CAD build for the part. Positions are in the model's coordinates, mm. A direction names the side the tool comes from. Round coordinates to 2 decimals unless told otherwise and drop trailing zeros. Write each loop counter-clockwise with the first axis right and the second up, starting at its lowest first coordinate (ties: lowest second). Pieces come first, ordered by that corner, then holes. Notation, with made-up numbers: (68.5, 23) -> (101.5, 23) arc R16 ccw to (101.5, 32) -> close; hole circle Ø8 at (88, 9). An arc over 180 degrees is marked (long way). Put each result on its own line as item: value. Start each with the question number.
1. Drill centre lines: line 1 (X direction, y = 7, z = -9); line 2 (Z direction, x = 2, y = 3.5); line 3 (Y direction, x = -4.5, z = 10). Where is each one in solid material? Low to high. Write a range as from..to.
2. Saw through at B-B on x = 5. List the corners of the cut face in (y, z).
3. 3-axis set-ups, long thin cutter, end or side, ignore diameter. For faces 4 (the flat face through (17, 0, -23)), 5 (the flat face through (13.79, 4, 2)), 6 (the flat face through (-32, -1, -26.874)), 7 (the flat face through (17, -1, 24.126)), 8 (the cylindrical face through (-34.64, -0.99, 24.73)): which of +Z, -Z, +X, -X, +Y, -Y reach the whole face in a straight line?
4. Saw through at C-C on z = -10.5. List the corners of the cut face in (x, y).
5. Pull direction Z, two halves, no side cores. Call faces 1 (the cylindrical face through (20.22, -0.986, 28.524)), 2 (the cylindrical face through (-34.64, -0.99, -26.27)), 3 (the cylindrical face through (20.22, -0.986, -22.476)): pulls with the +Z half, pulls with the -Z half, needs draft (parallel to the pull), parting line crosses it, or undercut.
6. Flat gauge pins, fed straight in: P1, Ø0.6, axis at x = -32, y = -0.5, coming from the -Z side; P2, Ø2, axis at x = 17.5, y = -0.5, coming from the +Z side; P3, Ø1.5, axis at y = -0.5, z = 4, coming from the -X side; P4, Ø4, axis at x = -32.71, z = 26.63, coming from the -Y side. Where does each tip first touch, or does it go through?
7. Saw through at A-A on y = 2.25. List the corners of the cut face in (x, z).
from build123d import *

# Parameters (mm, degrees)
SKETCH_1_W          = 46
SKETCH_1_H          = 62
EXTRUDE_1_DEPTH     = 8
SKETCH_2_W          = 42
SKETCH_2_H          = 58
CUT_EXTRUDE_1_DEPTH = 8
SKETCH_3_R          = 1.5
SKETCH_3_W          = 42
SKETCH_3_H          = 58
EXTRUDE_2_DEPTH     = 2


with BuildPart() as part:
    # 草图1 → 凸台-拉伸1 (new body)
    with BuildSketch(Plane(origin=(0, 0, 0), x_dir=(1, 0, 0), z_dir=(0, 1, 0))):
        with Locations((-7.20979021, -1.125874126)):
            Rectangle(SKETCH_1_W, SKETCH_1_H)
    extrude(amount=EXTRUDE_1_DEPTH)

    # 草图2 → 切除-拉伸1 (cut)
    with BuildSketch(Plane(origin=(0, 8, 0), x_dir=(1, 0, 0), z_dir=(0, 1, 0))):
        with Locations((-7.20979021, -1.125874126)):
            Rectangle(SKETCH_2_W, SKETCH_2_H)
    extrude(amount=-CUT_EXTRUDE_1_DEPTH, mode=Mode.SUBTRACT)

    # 草图3 → 凸台-拉伸2 (add)
    # profile 1 of 6: a face of its own
    with BuildSketch(Plane.XZ):
        with BuildLine():
            Line((-30.20979021, 24.125874126), (-30.20979021, 29.125874126))
            Line((-30.20979021, 29.125874126), (-33.20979021, 29.125874126))
            ThreePointArc((-33.20979021, 29.125874126), (-34.624003772, 28.540087688), (-35.20979021, 27.125874126))
            Line((-35.20979021, 27.125874126), (-35.20979021, 26.125874126))
            ThreePointArc((-35.20979021, 26.125874126), (-34.624003772, 24.711660564), (-33.20979021, 24.125874126))
            Line((-33.20979021, 24.125874126), (-30.20979021, 24.125874126))
        make_face()
        with Locations(Location((-32.70979021, 26.625874126, 0), (0, 0, 270))):
            Circle(SKETCH_3_R, mode=Mode.SUBTRACT)
    # profile 2 of 6: a face of its own
    with BuildSketch(Plane.XZ):
        Polygon((15.79020979, 32.125874126), (-30.20979021, 32.125874126), (-30.20979021, 29.125874126), (-30.20979021, 24.125874126), (-30.20979021, -21.874125874), (-30.20979021, -26.874125874), (-30.20979021, -29.874125874), (15.79020979, -29.874125874), (15.79020979, -26.874125874), (15.79020979, -21.874125874), (15.79020979, 24.125874126), (15.79020979, 29.125874126), align=None)
        with Locations((-7.20979021, 1.125874126)):
            Rectangle(SKETCH_3_W, SKETCH_3_H, mode=Mode.SUBTRACT)
    # profile 3 of 6: a face of its own
    with BuildSketch(Plane.XZ):
        with BuildLine():
            Line((18.79020979, 29.125874126), (15.79020979, 29.125874126))
            Line((15.79020979, 29.125874126), (15.79020979, 24.125874126))
            Line((15.79020979, 24.125874126), (18.79020979, 24.125874126))
            ThreePointArc((18.79020979, 24.125874126), (20.204423353, 24.711660564), (20.79020979, 26.125874126))
            Line((20.79020979, 26.125874126), (20.79020979, 27.125874126))
            ThreePointArc((20.79020979, 27.125874126), (20.204423353, 28.540087688), (18.79020979, 29.125874126))
        make_face()
        with Locations(Location((18.29020979, 26.625874126, 0), (0, 0, 270))):
            Circle(SKETCH_3_R, mode=Mode.SUBTRACT)
    # profile 4 of 6: a face of its own
    with BuildSketch(Plane.XZ):
        with BuildLine():
            Line((-30.20979021, -26.874125874), (-30.20979021, -21.874125874))
            Line((-30.20979021, -21.874125874), (-33.20979021, -21.874125874))
            ThreePointArc((-33.20979021, -21.874125874), (-34.624003772, -22.459912312), (-35.20979021, -23.874125874))
            Line((-35.20979021, -23.874125874), (-35.20979021, -24.874125874))
            ThreePointArc((-35.20979021, -24.874125874), (-34.624003772, -26.288339436), (-33.20979021, -26.874125874))
            Line((-33.20979021, -26.874125874), (-30.20979021, -26.874125874))
        make_face()
        with Locations(Location((-32.70979021, -24.374125874, 0), (0, 0, 270))):
            Circle(SKETCH_3_R, mode=Mode.SUBTRACT)
    # profile 5 of 6: a face of its own
    with BuildSketch(Plane.XZ):
        with BuildLine():
            Line((18.79020979, -21.874125874), (15.79020979, -21.874125874))
            Line((15.79020979, -21.874125874), (15.79020979, -26.874125874))
            Line((15.79020979, -26.874125874), (18.79020979, -26.874125874))
            ThreePointArc((18.79020979, -26.874125874), (20.204423353, -26.288339436), (20.79020979, -24.874125874))
            Line((20.79020979, -24.874125874), (20.79020979, -23.874125874))
            ThreePointArc((20.79020979, -23.874125874), (20.204423353, -22.459912312), (18.79020979, -21.874125874))
        make_face()
        with Locations(Location((18.29020979, -24.374125874, 0), (0, 0, 270))):
            Circle(SKETCH_3_R, mode=Mode.SUBTRACT)
    # profile 6 of 6: a face of its own
    with BuildSketch(Plane.XZ):
        with Locations((-7.20979021, 1.125874126)):
            Rectangle(SKETCH_3_W, SKETCH_3_H)
    extrude(amount=EXTRUDE_2_DEPTH)


solid = part.part
Return value:
1. line 1: x = -30.21..-28.21, 13.79..15.79
1. line 2: z = -29.87..-27.87, 30.13..32.13
1. line 3: y = -2..0
2. outline: (-2, -29.87) -> (8, -29.87) -> (8, -27.87) -> (0, -27.87) -> (0, 30.13) -> (8, 30.13) -> (8, 32.13) -> (-2, 32.13) -> close
3. face 4: +Z, -Z, +X, +Y
3. face 5: +Y
3. face 6: -Z, -X, +Y, -Y
3. face 7: +X, +Y, -Y
3. face 8: -X, +Y, -Y
4. outline: (-30.21, -2) -> (15.79, -2) -> (15.79, 8) -> (13.79, 8) -> (13.79, 0) -> (-28.21, 0) -> (-28.21, 8) -> (-30.21, 8) -> close
5. face 1: pulls with the +Z half
5. face 2: pulls with the -Z half
5. face 3: undercut
6. P1: stops at z = -26.87
6. P2: stops at z = 29.13
6. P3: stops at x = -30.21
6. P4: stops at y = -2
7. outline: (-30.21, -29.87) -> (15.79, -29.87) -> (15.79, 32.13) -> (-30.21, 32.13) -> close; hole (-28.21, -27.87) -> (13.79, -27.87) -> (13.79, 30.13) -> (-28.21, 30.13) -> close
